Geometry: final body of the model. Coordinates: model frame, mm. A direction names the side the tool comes from. Give positions to 0.01 mm unless a question says otherwise; leave off trailing zeros. Write each loop counter-clockwise with the first axis right and the second up, starting at its lowest first coordinate (ties: lowest second). Pieces come first, ordered by that corner, then holes. Notation, with made-up numbers: (-22, 75) -> (-4, 75) arc R12 cw to (-4, 95) -> close; hole circle Ø2 at (81, -11.75). An arc over 180 degrees is marked (long way). Answer in a Markdown table with one row per item. Add a question column.
from build123d import *

# Parameters (mm, degrees)
F0_W     = 144.4752
F0_H     = 63.5254
F1_DEPTH = 22.1742
F2_R     = 3.96875
F3_DEPTH = 22.1752
F5_DEPTH = 63.5264
F7_DEPTH = 15.7988
F9_DEPTH = 15.7988


with BuildPart() as f1:
    # F0 (on Front) → F1 (new body)
    with BuildSketch(Plane.XZ):
        Rectangle(F0_W, F0_H)
    extrude(amount=F1_DEPTH)

    # F2 (on face) → F3 (cut, through all)
    with BuildSketch(Plane.XZ.offset(22.1742)):
        with Locations((-57.3278, 22.2377)):
            Circle(F2_R)
        with Locations((-57.3278, -22.2377)):
            Circle(F2_R)
        with Locations((57.3278, -22.2377)):
            Circle(F2_R)
        with Locations((57.3278, 22.2377)):
            Circle(F2_R)
    extrude(amount=-F3_DEPTH, mode=Mode.SUBTRACT)

    # F4 (on face) → F5 (cut, through all)
    with BuildSketch(Plane(origin=(0, 0, -31.7627), x_dir=(1, 0, 0), z_dir=(0, 0, -1))):
        with BuildLine():
            ThreePointArc((30.9626, 0), (16.932301, 10.1335), (0, 13.716))
            ThreePointArc((0, 13.716), (-16.932301, 10.1335), (-30.9626, 0))
            Line((-30.9626, 0), (30.9626, 0))
        make_face()
    extrude(amount=-F5_DEPTH, mode=Mode.SUBTRACT)

    # F6 (on face) → F7 (cut)
    with BuildSketch(Plane(origin=(0, 0, 0), x_dir=(-1, 0, 0), z_dir=(0, 1, 0))):
        with BuildLine():
            ThreePointArc((-40.720254, 0), (-55.81231, -0.75452), (-40.7035, -0.50292))
            ThreePointArc((-40.7035, -0.50292), (-40.70769, -0.25132), (-40.720254, 0))
        make_face()
    extrude(amount=-F7_DEPTH, mode=Mode.SUBTRACT)

    # F8 (on face) → F9 (cut)
    with BuildSketch(Plane(origin=(0, 0, 0), x_dir=(-1, 0, 0), z_dir=(0, 1, 0))):
        with BuildLine():
            ThreePointArc((40.720254, 0), (48.0084, -8.05523), (55.8165, -0.50292))
            ThreePointArc((55.8165, -0.50292), (48.5116, 7.04939), (40.720254, 0))
        make_face()
    extrude(amount=-F9_DEPTH, mode=Mode.SUBTRACT)


solid = f1.part
Q1. Section C-C on z = -14. Return loops of the section in (x, y), and give its area (3 significant figures).
Q2. Section D-D on z = -3. Return loops of the section in (x, y), and give its area (3 significant figures).
Q3. Pull-direction query (Z, two-part tool) for faces 1 (the flat face through (56, 0, 0)), 2 (the flat face through (-1, -16, -31.763)), 3 (the cylindrical face through (61.1, -11.2, -21)); classes: +Z half, -Z half, draft (parallel to the pull), parting line (faces both ways), or undercut.
Q4. Contact query for a flat-ended pin moving along its axis: pin 1 Ø8 at (x, z) = (-19, -24.5) entering from +Y. Output: stop coordinate, or through.
Q5. Line query: probe 1 along X at (y, z) = (-17.5, 22.5); probe 2 along X at (y, z) = (-7.5, -24.5); probe 3 along X at (y, z) = (-6, -2). Output: solid intervals per line, ascending. Write a range as from..to.
Q6. Section B-B on y = -20.5. Return loops of the section in (x, z), and give its area (3 significant figures).
Q7. Section A-A on x = -48.26. Return loops of the section in (y, z), and give its area (3 significant figures).
Q8. Access query for faces 4 (the cylindrical face through (55.816, -7.789, -0.426)), 5 (the cylindrical face through (59.159, -11.242, 18.717)). Directions: +Z, -Z, +X, -X, +Y, -Y. A direction counts if a zero-diameter tool reaches every point of the face in a straight line with its end or side. Return the directions, or none.
Checks:
| question | item | result |
|---|---|---|
| 1 | outline | (-72.24, -22.17) -> (72.24, -22.17) -> (72.24, 0) -> (30.96, 0) arc R41.81 cw to (0, -13.72) arc R41.81 cw to (-30.96, 0) -> (-72.24, 0) -> close |
| 1 | area | 2,620 mm^2 |
| 2 | outline | (-72.24, -22.17) -> (72.24, -22.17) -> (72.24, 0) -> (55.39, 0) -> (55.39, -15.8) -> (41.13, -15.8) -> (41.13, 0) -> (30.96, 0) arc R41.81 cw to (0, -13.72) arc R41.81 cw to (-30.96, 0) -> (-41.13, 0) -> (-41.13, -15.8) -> (-55.39, -15.8) -> (-55.39, 0) -> (-72.24, 0) -> close |
| 2 | area | 2,170 mm^2 |
| 3 | face 1 | draft |
| 3 | face 2 | -Z half |
| 3 | face 3 | undercut |
| 4 | pin 1 | y = -6.82 |
| 5 | probe 1 | -72.24..-61.29, -53.37..53.37, 61.29..72.24 |
| 5 | probe 2 | -72.24..-60.59, -54.07..-21.93, 21.93..54.07, 60.59..72.24 |
| 5 | probe 3 | -72.24..-55.67, -40.85..-24.2, 24.2..40.85, 55.67..72.24 |
| 6 | outline | (-72.24, -31.76) -> (72.24, -31.76) -> (72.24, 31.76) -> (-72.24, 31.76) -> close; hole circle Ø7.94 at (-57.33, -22.24); hole circle Ø7.94 at (-57.33, 22.24); hole circle Ø7.94 at (57.33, -22.24); hole circle Ø7.94 at (57.33, 22.24) |
| 6 | area | 8,980 mm^2 |
| 7 | outline | (-22.17, -31.76) -> (0, -31.76) -> (0, -8.06) -> (-15.8, -8.06) -> (-15.8, 7.05) -> (0, 7.05) -> (0, 31.76) -> (-22.17, 31.76) -> close |
| 7 | area | 1,170 mm^2 |
| 8 | face 4 | +Y |
| 8 | face 5 | +Y, -Y |
